```python
from build123d import *

# Parameters (mm, degrees)
CIRPATTERN2_9_6_ANGLE   = 300
CIRPATTERN2_8_9_ANGLE   = 240
CIRPATTERN2_10_11_ANGLE = 300
CIRPATTERN2_7_13_ANGLE  = 240
CIRPATTERN2_6_15_ANGLE  = 180
CIRPATTERN2_5_17_ANGLE  = 180
CIRPATTERN2_4_19_ANGLE  = 120
CIRPATTERN2_2_21_ANGLE  = 60
CIRPATTERN2_3_23_ANGLE  = 120
CIRPATTERN2_25_ANGLE    = 60
THICKEN1_T2             = 1
BOSS_EXTRUDE1_DEPTH     = 1
BOSS_EXTRUDE2_DEPTH     = 1
SKETCH14_R              = 1
CUT_EXTRUDE1_DEPTH      = 5


with BuildPart() as body_1:
    # Sketch7 → Surface-Plane5: a flat surface bounded by the sketch
    with BuildSketch(Plane(origin=(-3.524717678, 1.028951947, -2.0349967), x_dir=(0.46535585521279793, -0.13573914338570603, -0.8746535388209896), z_dir=(0.8396091564737522, -0.24510260263935496, 0.484748572504189)), mode=Mode.PRIVATE) as surface_plane5_2_region:
        Polygon((2.623971283, -0.700846857), (-2.326779276, -1.400896074), (-5.009045109, 5.141691335), align=None)
    surface_plane5_2 = surface_plane5_2_region.sketch.faces()[0]
    # Sketch2 → Surface-Plane6: a flat surface bounded by the sketch
    with BuildSketch(Plane(origin=(0, 6.644630244, 0), x_dir=(1, 0, 0), z_dir=(0, 1, 0)), mode=Mode.PRIVATE) as surface_plane6_3_region:
        Polygon((-4.239819176, 2.650270431), (-4.415111108, -2.346655898), (-0.175291932, -4.996926329), (4.239819176, -2.650270431), (4.415111108, 2.346655898), (0.175291932, 4.996926329), align=None)
    surface_plane6_3 = surface_plane6_3_region.sketch.faces()[0]
    # Sketch6 → Surface-Plane4: a flat surface bounded by the sketch
    with BuildSketch(Plane(origin=(-2.489523341, -0.629773886, -0.087332357), x_dir=(0.07067634350540625, -0.14247920195053043, -0.9872712552689084), z_dir=(0.968901161979092, 0.24510260263935799, 0.03398900550145962)), mode=Mode.PRIVATE) as surface_plane4_4_region:
        Polygon((4.098319079, 1.265627187), (1.370159284, 7.789210875), (-3.575551438, 7.054401069), align=None)
    surface_plane4_4 = surface_plane4_4_region.sketch.faces()[0]
    # Sketch6 → Surface-Plane4: a flat surface bounded by the sketch
    with BuildSketch(Plane(origin=(-2.489523341, -0.629773886, -0.087332357), x_dir=(0.07067634350540625, -0.14247920195053043, -0.9872712552689084), z_dir=(0.968901161979092, 0.24510260263935799, 0.03398900550145962)), mode=Mode.PRIVATE) as surface_plane4_5_region:
        Polygon((4.098319079, 1.265627187), (1.370159284, 7.789210875), (-3.575551438, 7.054401069), align=None)
    surface_plane4_5 = surface_plane4_5_region.sketch.faces()[0]
    # CirPattern2 9: a copy of that surface (a pattern of surface bodies)
    cirpattern2_9_6 = surface_plane4_5.rotate(Axis((0, 0, 0), (0, 1, 0)), CIRPATTERN2_9_6_ANGLE)
    # Sketch1 → Surface-Plane7: a flat surface bounded by the sketch
    with BuildSketch(Plane(origin=(0, 0, 0), x_dir=(1, 0, 0), z_dir=(0, 1, 0)), mode=Mode.PRIVATE) as surface_plane7_7_region:
        Polygon((5, 0), (2.5, 4.330127019), (-2.5, 4.330127019), (-5, 0), (-2.5, -4.330127019), (2.5, -4.330127019), align=None)
    surface_plane7_7 = surface_plane7_7_region.sketch.faces()[0]
    # Sketch7 → Surface-Plane5: a flat surface bounded by the sketch
    with BuildSketch(Plane(origin=(-3.524717678, 1.028951947, -2.0349967), x_dir=(0.46535585521279793, -0.13573914338570603, -0.8746535388209896), z_dir=(0.8396091564737522, -0.24510260263935496, 0.484748572504189)), mode=Mode.PRIVATE) as surface_plane5_8_region:
        Polygon((2.623971283, -0.700846857), (-2.326779276, -1.400896074), (-5.009045109, 5.141691335), align=None)
    surface_plane5_8 = surface_plane5_8_region.sketch.faces()[0]
    # CirPattern2 8: a copy of that surface (a pattern of surface bodies)
    cirpattern2_8_9 = surface_plane5_8.rotate(Axis((0, 0, 0), (0, 1, 0)), CIRPATTERN2_8_9_ANGLE)
    # Sketch7 → Surface-Plane5: a flat surface bounded by the sketch
    with BuildSketch(Plane(origin=(-3.524717678, 1.028951947, -2.0349967), x_dir=(0.46535585521279793, -0.13573914338570603, -0.8746535388209896), z_dir=(0.8396091564737522, -0.24510260263935496, 0.484748572504189)), mode=Mode.PRIVATE) as surface_plane5_10_region:
        Polygon((2.623971283, -0.700846857), (-2.326779276, -1.400896074), (-5.009045109, 5.141691335), align=None)
    surface_plane5_10 = surface_plane5_10_region.sketch.faces()[0]
    # CirPattern2 10: a copy of that surface (a pattern of surface bodies)
    cirpattern2_10_11 = surface_plane5_10.rotate(Axis((0, 0, 0), (0, 1, 0)), CIRPATTERN2_10_11_ANGLE)
    # Sketch6 → Surface-Plane4: a flat surface bounded by the sketch
    with BuildSketch(Plane(origin=(-2.489523341, -0.629773886, -0.087332357), x_dir=(0.07067634350540625, -0.14247920195053043, -0.9872712552689084), z_dir=(0.968901161979092, 0.24510260263935799, 0.03398900550145962)), mode=Mode.PRIVATE) as surface_plane4_12_region:
        Polygon((4.098319079, 1.265627187), (1.370159284, 7.789210875), (-3.575551438, 7.054401069), align=None)
    surface_plane4_12 = surface_plane4_12_region.sketch.faces()[0]
    # CirPattern2 7: a copy of that surface (a pattern of surface bodies)
    cirpattern2_7_13 = surface_plane4_12.rotate(Axis((0, 0, 0), (0, 1, 0)), CIRPATTERN2_7_13_ANGLE)
    # Sketch7 → Surface-Plane5: a flat surface bounded by the sketch
    with BuildSketch(Plane(origin=(-3.524717678, 1.028951947, -2.0349967), x_dir=(0.46535585521279793, -0.13573914338570603, -0.8746535388209896), z_dir=(0.8396091564737522, -0.24510260263935496, 0.484748572504189)), mode=Mode.PRIVATE) as surface_plane5_14_region:
        Polygon((2.623971283, -0.700846857), (-2.326779276, -1.400896074), (-5.009045109, 5.141691335), align=None)
    surface_plane5_14 = surface_plane5_14_region.sketch.faces()[0]
    # CirPattern2 6: a copy of that surface (a pattern of surface bodies)
    cirpattern2_6_15 = surface_plane5_14.rotate(Axis((0, 0, 0), (0, 1, 0)), CIRPATTERN2_6_15_ANGLE)
    # Sketch6 → Surface-Plane4: a flat surface bounded by the sketch
    with BuildSketch(Plane(origin=(-2.489523341, -0.629773886, -0.087332357), x_dir=(0.07067634350540625, -0.14247920195053043, -0.9872712552689084), z_dir=(0.968901161979092, 0.24510260263935799, 0.03398900550145962)), mode=Mode.PRIVATE) as surface_plane4_16_region:
        Polygon((4.098319079, 1.265627187), (1.370159284, 7.789210875), (-3.575551438, 7.054401069), align=None)
    surface_plane4_16 = surface_plane4_16_region.sketch.faces()[0]
    # CirPattern2 5: a copy of that surface (a pattern of surface bodies)
    cirpattern2_5_17 = surface_plane4_16.rotate(Axis((0, 0, 0), (0, 1, 0)), CIRPATTERN2_5_17_ANGLE)
    # Sketch7 → Surface-Plane5: a flat surface bounded by the sketch
    with BuildSketch(Plane(origin=(-3.524717678, 1.028951947, -2.0349967), x_dir=(0.46535585521279793, -0.13573914338570603, -0.8746535388209896), z_dir=(0.8396091564737522, -0.24510260263935496, 0.484748572504189)), mode=Mode.PRIVATE) as surface_plane5_18_region:
        Polygon((2.623971283, -0.700846857), (-2.326779276, -1.400896074), (-5.009045109, 5.141691335), align=None)
    surface_plane5_18 = surface_plane5_18_region.sketch.faces()[0]
    # CirPattern2 4: a copy of that surface (a pattern of surface bodies)
    cirpattern2_4_19 = surface_plane5_18.rotate(Axis((0, 0, 0), (0, 1, 0)), CIRPATTERN2_4_19_ANGLE)
    # Sketch7 → Surface-Plane5: a flat surface bounded by the sketch
    with BuildSketch(Plane(origin=(-3.524717678, 1.028951947, -2.0349967), x_dir=(0.46535585521279793, -0.13573914338570603, -0.8746535388209896), z_dir=(0.8396091564737522, -0.24510260263935496, 0.484748572504189)), mode=Mode.PRIVATE) as surface_plane5_20_region:
        Polygon((2.623971283, -0.700846857), (-2.326779276, -1.400896074), (-5.009045109, 5.141691335), align=None)
    surface_plane5_20 = surface_plane5_20_region.sketch.faces()[0]
    # CirPattern2 2: a copy of that surface (a pattern of surface bodies)
    cirpattern2_2_21 = surface_plane5_20.rotate(Axis((0, 0, 0), (0, 1, 0)), CIRPATTERN2_2_21_ANGLE)
    # Sketch6 → Surface-Plane4: a flat surface bounded by the sketch
    with BuildSketch(Plane(origin=(-2.489523341, -0.629773886, -0.087332357), x_dir=(0.07067634350540625, -0.14247920195053043, -0.9872712552689084), z_dir=(0.968901161979092, 0.24510260263935799, 0.03398900550145962)), mode=Mode.PRIVATE) as surface_plane4_22_region:
        Polygon((4.098319079, 1.265627187), (1.370159284, 7.789210875), (-3.575551438, 7.054401069), align=None)
    surface_plane4_22 = surface_plane4_22_region.sketch.faces()[0]
    # CirPattern2 3: a copy of that surface (a pattern of surface bodies)
    cirpattern2_3_23 = surface_plane4_22.rotate(Axis((0, 0, 0), (0, 1, 0)), CIRPATTERN2_3_23_ANGLE)
    # Sketch6 → Surface-Plane4: a flat surface bounded by the sketch
    with BuildSketch(Plane(origin=(-2.489523341, -0.629773886, -0.087332357), x_dir=(0.07067634350540625, -0.14247920195053043, -0.9872712552689084), z_dir=(0.968901161979092, 0.24510260263935799, 0.03398900550145962)), mode=Mode.PRIVATE) as surface_plane4_24_region:
        Polygon((4.098319079, 1.265627187), (1.370159284, 7.789210875), (-3.575551438, 7.054401069), align=None)
    surface_plane4_24 = surface_plane4_24_region.sketch.faces()[0]
    # CirPattern2: a copy of that surface (a pattern of surface bodies)
    cirpattern2_25 = surface_plane4_24.rotate(Axis((0, 0, 0), (0, 1, 0)), CIRPATTERN2_25_ANGLE)
    # Surface-Knit1: the surfaces knitted into one
    surface_knit1_1 = Shell(Face.sew_faces(surface_plane5_2.faces() + surface_plane6_3.faces() + surface_plane4_4.faces() + cirpattern2_9_6.faces() + surface_plane7_7.faces() + cirpattern2_8_9.faces() + cirpattern2_10_11.faces() + cirpattern2_7_13.faces() + cirpattern2_6_15.faces() + cirpattern2_5_17.faces() + cirpattern2_4_19.faces() + cirpattern2_2_21.faces() + cirpattern2_3_23.faces() + cirpattern2_25.faces())[0])
    add(Solid.thicken(surface_knit1_1, -THICKEN1_T2))

    # Sketch12 → Boss-Extrude1 (add)
    with BuildSketch(Plane(origin=(0, 6.644630244, 0), x_dir=(1, 0, 0), z_dir=(0, 1, 0))):
        Polygon((0.175291932, 4.996926329), (-4.239819176, 2.650270431), (-4.415111108, -2.346655898), (-0.175291932, -4.996926329), (4.239819176, -2.650270431), (4.415111108, 2.346655898), align=None)
    extrude(amount=BOSS_EXTRUDE1_DEPTH)

    # Sketch13 → Boss-Extrude2 (add)
    with BuildSketch(Plane.XZ):
        Polygon((5, 0), (2.5, 4.330127019), (-2.5, 4.330127019), (-5, 0), (-2.5, -4.330127019), (2.5, -4.330127019), align=None)
    extrude(amount=BOSS_EXTRUDE2_DEPTH)

    # Sketch14 → Cut-Extrude1 (cut)
    with BuildSketch(Plane.XZ.offset(1)):
        with Locations(Location((0, 0, 0), (0, 0, 270))):
            Circle(SKETCH14_R)
    extrude(amount=-CUT_EXTRUDE1_DEPTH, mode=Mode.SUBTRACT)


solid = body_1.part
```
Verification items for the finished model (mm, model axes). A direction names the side the tool comes from. Coordinates: 2 decimals unless noted, no trailing zeros. Loops run counter-clockwise (first coordinate to the right, second up) from the corner with the lowest first, then second, coordinate; pieces in that order, holes last. Notation, with made-up numbers: (-39.5, 15) - (-19.5, 15) arc R23 cw to (-19.5, 47) - close; hole circle Ø2 at (44, -34). An arc over 180 degrees is marked (long way). Answer as a JSON object with one key per item and string values.
(1) Mould release check, pull along X, two halves, no side actions. Record for faces 1 (the flat face through (2.597, 2.339, -2.979)), 2 (the flat face through (1, 1, -1)), 3 (the flat face through (-2.597, 2.339, 2.979)): pulls with the +X half, pulls with the -X half, needs draft (parallel to the pull), parting line crosses it, or undercut.
Response:
{"face 1": "pulls with the +X half", "face 2": "undercut", "face 3": "pulls with the -X half"}
(2) Cross-section at D-D, the plane x = -0.5. Record the boundary of the cut face in (y, z).
Response:
{"outline": "(-1, -4.33) - (0, -4.33) - (2.96, -3.58) - (6.64, -4.64) - (7.64, -4.64) - (7.64, 4.79) - (6.64, 4.79) - (6.2, 4.66) - (5.72, 4.9) - (1.97, 3.83) - (0, 4.33) - (-1, 4.33) - (-1, 0.87) - (1, 0.87) - (1, 3.05) - (2.23, 2.74) - (4.59, 3.41) - (5.14, 3.13) - (5.64, 3.28) - (5.64, -3.18) - (3.21, -2.49) - (1, -3.05) - (1, -0.87) - (-1, -0.87) - close"}
(3) Go/stop test with flat-tipped pins: pin 1 Ø5 at (x, y) = (-2.5, 1.5) entering from -Z; pin 2 Ø3 at (y, z) = (6, 2) entering from +X; pin 3 Ø0.8 at (x, y) = (1, -0.5) entering from +Z. Record where each tip stops, or that it passes through.
Response:
{"pin 1": "stops at z = -4.33", "pin 2": "stops at x = 4.31", "pin 3": "stops at z = 4.33"}
(4) Scan lines: line 1 along Y through (x, z) = (-1, 0.25); line 2 along X through (y, z) = (1.25, -1); line 3 along Z through (x, y) = (-2.75, 2.75). Record each from-to range of solid material in increasing order.
Response:
{"line 1": "y = -1 to 1, 5.64 to 7.64", "line 2": "x = -4.06 to -2.87, 2.87 to 4.06", "line 3": "z = -3.63 to -0.44, 1.01 to 2.51"}
(5) Cross-section at A-A, the plane x = 2. Record the boundary of the cut face in (y, z).
Response:
{"outline": "(-1, -4.33) - (0, -4.33) - (0.49, -4.21) - (1.43, -4.47) - (4.13, -3.11) - (6.64, -3.86) - (7.64, -3.86) - (7.64, 3.84) - (6.64, 3.84) - (4.44, 3.21) - (0, 4.33) - (-1, 4.33) - close; hole (1, -2.63) - (3.08, -1.58) - (5.64, -2.34) - (5.64, 2.39) - (4.69, 2.11) - (1.89, 2.82) - (1.81, 2.22) - (1, 2.63) - close"}
(6) Cross-section at B-B, the plane z = -0.5. Record the boundary of the cut face in (x, y).
Response:
{"outline": "(-4.71, -1) - (-0.87, -1) - (-0.87, 1) - (-3.23, 1) - (-2.49, 3.52) - (-3.03, 5.64) - (3.07, 5.64) - (2.78, 4.52) - (3.4, 2.4) - (3.04, 1.65) - (3.23, 1) - (0.87, 1) - (0.87, -1) - (4.71, -1) - (4.71, 0) - (4.52, 0.66) - (4.88, 1.42) - (3.89, 4.81) - (4.35, 6.64) - (4.35, 7.64) - (-4.32, 7.64) - (-4.32, 6.64) - (-3.6, 3.81) - (-4.71, 0) - close"}
(7) Access from +Z, -Z, +X, -X, +Y, -Y to the whole of each face (thin tool, end or side, straight path). Record for faces 4 (the flat face through (-3.88, 2.34, -0.76)), 5 (the flat face through (3.88, 2.34, 0.76)), 6 (the flat face through (3.73, -0.49, -2.2)).
Response:
{"face 4": "-Z, -X", "face 5": "+Z, +X", "face 6": "-Z, +X, -Y"}
(8) Cross-section at C-C, the plane y = 2.25. Record the boundary of the cut face in (x, z), then the cut area to 3 significant figures.
Response:
{"outline": "(-4.8, 0.79) - (-3.15, -2.07) - (-3.09, -3.76) - (0.22, -3.76) - (1.71, -4.56) - (3.37, -1.69) - (4.8, -0.79) - (3.15, 2.07) - (3.09, 3.76) - (-0.22, 3.76) - (-1.71, 4.56) - (-3.37, 1.69) - close; hole (-3.41, 0.45) - (-2.13, -1.78) - (-2.09, -2.73) - (0.47, -2.73) - (1.32, -3.18) - (2.6, -0.95) - (3.41, -0.45) - (2.13, 1.78) - (2.09, 2.73) - (-0.47, 2.73) - (-1.32, 3.18) - (-2.6, 0.95) - close", "area": "26.4 mm²"}
